from build123d import *

# Parameters (mm, degrees)
F0_W     = 55
F0_H     = 5
F1_DEPTH = 35
F3_D     = 12


with BuildPart() as f1:
    # F0 (on Top) → F1 (new body)
    with BuildSketch(Plane.XY):
        Polygon((0, -40), (0, 0), (-5, 0), (-5, -45), (0, -45), align=None)
        Polygon((-5, 0), (0, 0), (0, 40), (0, 45), (-5, 45), align=None)
        with Locations((27.5, 42.5)):
            Rectangle(F0_W, F0_H)
        with Locations((27.5, -42.5)):
            Rectangle(F0_W, F0_H)
    extrude(amount=F1_DEPTH)

    # F3 (through all)
    with Locations(Plane(origin=(0, 45, 0), x_dir=(-1, 0, 0), z_dir=(0, 1, 0))):
        with Locations((-27, 17.614661)):
            Hole(F3_D / 2)


solid = f1.part
Input: part model. Units: mm. Frame: model coordinates. A direction names the side the tool comes from. Coordinates: 2 decimals unless noted, no trailing zeros. Loops run counter-clockwise (first coordinate to the right, second up) from the corner with the lowest first, then second, coordinate; pieces in that order, holes last. Notation, with made-up numbers: (36, -34.5) - (76, -34.5) arc R23 ccw to (76, -13.5) - close; hole circle Ø4 at (-6.75, 8.25). An arc over 180 degrees is marked (long way). Answer in a Markdown table with one row per item. Add a question column.
Item 1: Section query D-D on y = 9.5. Return the cut outline in (x, z).
Item 2: Line query: line 1 along Z through (x, y) = (27, 42.5); line 2 along Y through (x, z) = (8, 3); line 3 along X through (y, z) = (-25, 30). Output: solid intervals per line, ascending. Write a range as [from, to].
Item 3: Mould query, pull axis X, two halves, no side actions, for faces 3 (the cylindrical face through (22.24, -42.54, 13.96)), 4 (the flat face through (-2, 4, 0)), 5 (the flat face through (0, -1, 17)). Classes: released by +X, released by -X, zero draft, split by the parting line, or undercut.
Item 4: Section query B-B on x = 17. Return the cut outline in (y, z).
Item 5: Access query for faces 1 (the flat face through (33.2, 40, 17.3)), 2 (the flat face through (-5, 1, 17)). Directions: +Z, -Z, +X, -X, +Y, -Y. A direction counts if a zero-diameter tool reaches every point of the face in a straight line with its end or side. Return the directions, or none.
Item 6: Section query C-C on z = 15.5. Return the cut outline in (x, y) (3 decimals).
Item 7: Section query A-A on x = 27. Return the cut outline in (y, z).
Item 8: Contact query for a flat-ended pin moving along its axis: P1, Ø10, axis at y = -31.5, z = 14, coming from the +X side. Output: stop coordinate, or through.
Recorded:
| question | item | result |
|---|---|---|
| 1 | outline | (-5, 0) - (0, 0) - (0, 35) - (-5, 35) - close |
| 2 | line 1 | [0, 11.61], [23.61, 35] |
| 2 | line 2 | [-45, -40], [40, 45] |
| 2 | line 3 | [-5, 0] |
| 3 | face 3 | undercut |
| 3 | face 4 | zero draft |
| 3 | face 5 | released by +X |
| 4 | outline | (-45, 0) - (-40, 0) - (-40, 35) - (-45, 35) - close; (40, 0) - (45, 0) - (45, 35) - (40, 35) - close |
| 5 | face 1 | +Z, -Z, +X |
| 5 | face 2 | +Z, -Z, -X, +Y, -Y |
| 6 | outline | (-5, -45) - (21.385, -45) - (21.385, -40) - (0, -40) - (0, 40) - (21.385, 40) - (21.385, 45) - (-5, 45) - close; (32.615, -45) - (55, -45) - (55, -40) - (32.615, -40) - close; (32.615, 40) - (55, 40) - (55, 45) - (32.615, 45) - close |
| 7 | outline | (-45, 0) - (-40, 0) - (-40, 11.61) - (-45, 11.61) - close; (-45, 23.61) - (-40, 23.61) - (-40, 35) - (-45, 35) - close; (40, 0) - (45, 0) - (45, 11.61) - (40, 11.61) - close; (40, 23.61) - (45, 23.61) - (45, 35) - (40, 35) - close |
| 8 | P1 | x = 0 |
